```python
from build123d import *

# Parameters (mm, degrees)
F1_DEPTH = 30
F2_R     = 5
F3_DEPTH = 12.7077577636
F5_DEPTH = 15.0035852566
F8_DEPTH = 8
F11_R    = 5


# Not quite as in the source:
# - a pattern or mirror of a feature is missing from the dataset's text; its kind, count and spacing are read off the source's solid
# - the program builds the solid bodies; features that only make, move or delete a surface that nothing else refers to are left out


with BuildPart() as f1:
    # F0 (on Front) → F1 (new body, symmetric)
    with BuildSketch(Plane.XZ):
        Polygon((-51.0283857584, 15.0035852566), (-51.0283857584, 0), (0, 0), (0, 48.1919869781), (-12.7077577636, 48.1919869781), (-12.7077577636, 15.0035852566), align=None)
    extrude(amount=F1_DEPTH, both=True)

    # F2 (on face) → F3 (cut, through all)
    with BuildSketch(Plane.YZ):
        with Locations((0, 35.1077616215)):
            Circle(F2_R)
    extrude(amount=-F3_DEPTH, mode=Mode.SUBTRACT)

    # F4 (on face) → F5 (cut, through all)
    with BuildSketch(Plane.XY.offset(15.0035852566)):
        with BuildLine():
            ThreePointArc((-42.0283857584, -5), (-38.4928518525, -3.5355339059), (-37.0283857584, 0))
            ThreePointArc((-37.0283857584, 0), (-38.4928518525, 3.5355339059), (-42.0283857584, 5))
            ThreePointArc((-42.0283857584, 5), (-47.0283857584, 0), (-42.0283857584, -5))
        make_face()
        with BuildLine():
            ThreePointArc((-42.0283857584, -5), (-47.0283857584, 0), (-42.0283857584, 5))
            Line((-42.0283857584, 5), (-51.0283857584, 5))
            Line((-51.0283857584, 5), (-51.0283857584, -5))
            Line((-51.0283857584, -5), (-42.0283857584, -5))
        make_face()
    extrude(amount=-F5_DEPTH, mode=Mode.SUBTRACT)

    # F7 (on offset) → F8 (join)
    with BuildSketch(Plane.XZ.offset(18)):
        Polygon((-12.7077577636, 39.0035852566), (-24.7077577636, 15.0035852566), (-12.7077577636, 15.0035852566), align=None)
    f8 = extrude(amount=F8_DEPTH)

    # F8_copies: F8 across plane
    add(f8.mirror(Plane.ZX))

    # F11
    f11_edges = [f1.edges().sort_by_distance(p)[0] for p in [
        (-6.353879, 30, 48.191987),
        (-6.353879, -30, 48.191987),
    ]]
    fillet(f11_edges, radius=F11_R)


solid = f1.part
```
Could you check a few things on this model? Use its own coordinates, in mm. A direction names the side the tool comes from. Round coordinates to 2 decimals unless told otherwise and drop trailing zeros. Loops run counter-clockwise (first coordinate to the right, second up) from the corner with the lowest first, then second, coordinate; pieces in that order, holes last.
Q1. I want a section at C-C (z = 9). Write out the boundary of the cut face in (x, y), and give its area (3 significant figures).
Q2. I want a section at B-B (y = -2). Write out the boundary of the cut face in (x, z), and give its area (3 significant figures).
Q3. Please list where these lines run through material, in increasing order: L1, parallel to Z at x = -7, y = 0; L2, parallel to Y at x = -43.5, z = 5; L3, parallel to Z at x = -36, y = 17.5.
Q4. For P1, Ø11.5, axis at y = 0, z = 35.11, coming from the -X side; P2, Ø19, axis at x = -28.5, y = 2, coming from the +Z side; P3, Ø13, axis at x = -20.5, z = 27.5, coming from the +Y side; P4, Ø12, axis at x = -24, z = 31.5, coming from the -Y side, each with a flat end and sliding along its axis, tell me the tip position at first contact or that it passes through.
Q5. Thinking about a two-plate mould opening in Y: for faces 1 (the cylindrical face through (-6.44, 28.57, 46.69)), 2 (the flat face through (-20, -30, 12)), 3 (the cylindrical face through (-6.265, 2.688, 39.324)), 4 (the flat face through (-12.708, 0, 28)), which applies, pulls with the +Y half, pulls with the -Y half, needs draft (parallel to the pull), parting line crosses it, or undercut?
Q6. On a 3-axis mill with a long thin cutter (end or side, diameter ignored), from which of +Z, -Z, +X, -X, +Y, -Y can I reach the whole of each face in a straight line? I mean faces 5 (the flat face through (-51.028, 17, 8)), 6 (the flat face through (-16, -18, 22)), 7 (the flat face through (-16, 26, 22)), 8 (the flat face through (-46, 5, 8)), 9 (the flat face through (-16, -26, 22)). Say none if no direction works.
Q7. I want a section at D-D (z = 31.5). Write out the boundary of the cut face in (x, y), and give its area (3 significant figures).
Q8. I want a section at A-A (y = -22). Write out the boundary of the cut face in (x, z), and give its area (3 significant figures).
Answer below:
1. outline: (-51.03, -30) - (0, -30) - (0, 30) - (-51.03, 30) - (-51.03, 5) - (-42.03, 5) arc R5 cw to (-42.03, -5) - (-51.03, -5) - close
1. area: 2,930 mm2
2. outline: (-37.45, 0) - (0, 0) - (0, 30.53) - (-12.71, 30.53) - (-12.71, 15) - (-37.45, 15) - close; (-12.71, 39.69) - (0, 39.69) - (0, 48.19) - (-12.71, 48.19) - close
2. area: 867 mm2
3. L1: z = 0 to 30.11, 40.11 to 48.19
3. L2: y = -30 to -5, 5 to 30
3. L3: z = 0 to 15
4. P1: stops at x = -12.71
4. P2: stops at z = 15
4. P3: stops at y = 26
4. P4: passes through
5. face 1: pulls with the +Y half
5. face 2: pulls with the -Y half
5. face 3: undercut
5. face 4: undercut
6. face 5: +Z, -Z, -X, +Y, -Y
6. face 6: +Z, -X
6. face 7: +Z, -X, +Y
6. face 8: +Z, -Z, -X
6. face 9: +Z, -X, -Y
7. outline: (-16.46, -26) - (-12.71, -26) - (-12.71, -30) - (0, -30) - (0, -3.46) - (-12.71, -3.46) - (-12.71, -18) - (-16.46, -18) - close; (-16.46, 18) - (-12.71, 18) - (-12.71, 3.46) - (0, 3.46) - (0, 30) - (-12.71, 30) - (-12.71, 26) - (-16.46, 26) - close
7. area: 735 mm2
8. outline: (-51.03, 0) - (0, 0) - (0, 48.19) - (-12.71, 48.19) - (-12.71, 39) - (-24.71, 15) - (-51.03, 15) - close
8. area: 1,330 mm2
